from build123d import *

# Parameters (mm, degrees)
CUT_EXTRUDE2_DEPTH = 1.02


with BuildPart() as part:
    # Sketch14 → Revolve1 (revolve)
    with BuildSketch(Plane(origin=(0, 0, 0), x_dir=(0, 0, -1), z_dir=(1, 0, 0)), mode=Mode.PRIVATE) as revolve1_sk:
        Polygon((-8.35, 0), (-8.35, 3), (-8.25, 3), (-6.75, 1.5), (-6.65, 1.5), (6.275, 1.5), (6.65, 1.125), (6.65, 0), align=None)
    revolve(revolve1_sk.sketch.rotate(Axis((0, 0, -6.65), (0, 0, 1)), 90), axis=Axis((0, 0, -6.65), (0, 0, 1)))

    # Sketch5 → Cut-Extrude2 (cut)
    with BuildSketch(Plane.XY.offset(8.35)):
        Polygon((0, -1.154700538), (1, -0.577350269), (1, 0.577350269), (0, 1.154700538), (-1, 0.577350269), (-1, -0.577350269), align=None)
    extrude(amount=-CUT_EXTRUDE2_DEPTH, mode=Mode.SUBTRACT)


solid = part.part
Input: part model. Units: mm. Frame: model coordinates. A direction names the side the tool comes from. Coordinates: 2 decimals unless noted, no trailing zeros. Loops run counter-clockwise (first coordinate to the right, second up) from the corner with the lowest first, then second, coordinate; pieces in that order, holes last.
Q1. Cut plane A-A (y = 0). Output: boundary loops of the cut face in (x, z) (3 decimals), then the cut area to 3 significant figures.
Q2. Contact query for flat-ended pins moving along their axis: pin 1 (0.8 mm diameter, centred on y = 0, z = 8, fed in from +X); pin 2 (3 mm diameter, centred on x = 1.5, z = 4.5, fed in from -Y). Output: stop coordinate, or through.
Q3. Material intervals for line 1 (Y direction, x = 0.35, z = 7.75); line 2 (Z direction, x = -0.8, y = -1.2); line 3 (Z direction, x = -0.3, y = -2.5), sorted ascending.
Q4. Cut plane B-B (z = -0.5). Output: boundary loops of the cut face in (x, y).
Q5. Set-up query: faces 4 (the face through (1.3, 0, 8.35)), 5 (the face through (0.49, -0.87, 7.85)). Return all of +Z, -Z, +X, -X, +Y, -Y with unobstructed straight access to the full face (end or side cutting, diameter ignored); none if empty.
Q6. Draft query along Y for faces 1 (the face through (0, 0, -6.65)), 2 (the face through (-1.43, -0.45, 0.33)), 3 (the face through (-1, 0, 8)). Return one class per face: +Y half, -Y half, draft (parallel to the pull), parting line (faces both ways), or undercut.
Working result:
1. outline: (-3, 8.25) - (-1.5, 6.75) - (-1.5, -6.275) - (-1.125, -6.65) - (1.125, -6.65) - (1.5, -6.275) - (1.5, 6.75) - (3, 8.25) - (3, 8.35) - (1, 8.35) - (1, 7.33) - (-1, 7.33) - (-1, 8.35) - (-3, 8.35) - close
1. area: 45.4 mm2
2. pin 1: stops at x = 3
2. pin 2: stops at y = -1.5
3. line 1: y = -2.48 to -0.95, 0.95 to 2.48
3. line 2: z = -6.33 to 8.35
3. line 3: z = 7.77 to 8.35
4. outline: circle Ø3 at (0, 0)
5. face 4: +Z, +X, -X, +Y, -Y
5. face 5: +Z
6. face 1: draft
6. face 2: parting line
6. face 3: undercut
